Source: CAD feature listing. Evaluate the final solid. Frame: model axes, mm. Give positions to 0.01 mm unless a question says otherwise; leave off trailing zeros. Order: outer loops, then holes, each group sorted by start corner. A loop starts at its lowest first (then second) coordinate and runs counter-clockwise, first axis right, second up. Notation, with made-up numbers: M 74,11.5 L 123,11.5 A11 ccw 123,21.5 Z; hole C 78,13 d6. An arc over 180 degrees is marked long. Use CSV: the item, a comma, the result in double quotes. Start each with the question number.
1. Section query C-C, the plane y = -3.5. Return the cut outline in (x, z), plus the area to 3 significant figures.
2. Section query D-D, the plane x = -20. Return the cut outline in (y, z).
3. Line query: line 1 along X through (y, z) = (-1.25, 0.35); line 2 along Y through (x, z) = (30, 1.55); line 3 along X through (y, z) = (-0.5, 2.9). Output: solid intervals per line, ascending. Write a range as [from, to].
4. Pin query (flat end, axial travel): P1, Ø1.5, axis at y = 2, z = 1.5, coming from the -X side; P2, Ø2.5, axis at x = -20, y = 0, coming from the -Z side. Return the tip coordinate at first contact, or that it passes through.
5. Section query B-B, the plane z = 1.3. State how many separate pieces and enclosed holes the cut face has, plus the area to 3 significant figures.
6. Section query A-A, the plane x = 30. Return the cut outline in (y, z).
from build123d import *

# Parameters (mm, degrees)
SKETCH_1_W      = 60
SKETCH_1_H      = 12
SKETCH_1_R      = 1.5
EXTRUDE_1_DEPTH = 4
FILLET_1_R      = 6


with BuildPart() as part:
    # 草图1 → 凸台-拉伸1 (new body)
    with BuildSketch(Plane.XY):
        with Locations((5, 0)):
            Rectangle(SKETCH_1_W, SKETCH_1_H)
        with Locations((-20, 0)):
            Circle(SKETCH_1_R, mode=Mode.SUBTRACT)
        with Locations((30, 0)):
            Circle(SKETCH_1_R, mode=Mode.SUBTRACT)
    extrude(amount=EXTRUDE_1_DEPTH)

    # 圆角1
    fillet_1_edges = [part.edges().sort_by_distance(p)[0] for p in [
        (-25, -6, 2),
        (-25, 6, 2),
    ]]
    fillet(fillet_1_edges, radius=FILLET_1_R - 0.0001)  # a hair under: the kernel refuses the full size


solid = part.part
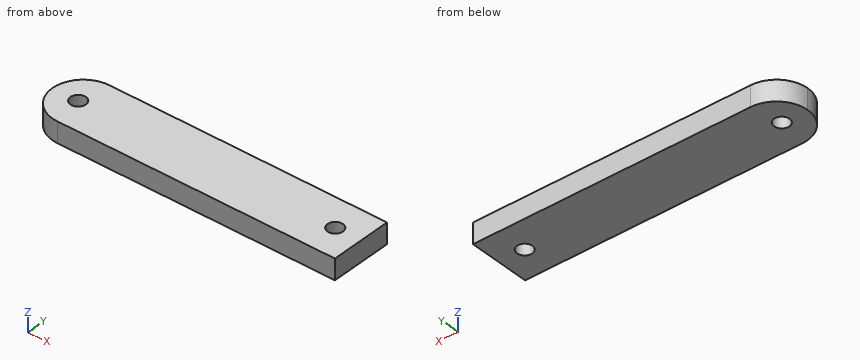
Result set:
1,outline,"M -23.87,0 L 35,0 L 35,4 L -23.87,4 Z"
1,area,"235 mm2"
2,outline,"M -5.92,0 L -1.5,0 L -1.5,4 L -5.92,4 Z; M 1.5,0 L 5.92,0 L 5.92,4 L 1.5,4 Z"
3,line 1,"[-24.87, -20.83], [-19.17, 29.17], [30.83, 35]"
3,line 2,"[-6, -1.5], [1.5, 6]"
3,line 3,"[-24.98, -21.41], [-18.59, 28.59], [31.41, 35]"
4,P1,"x = -24.87"
4,P2,"through"
5,separate pieces,"1"
5,enclosed holes,"2"
5,area,"690 mm2"
6,outline,"M -6,0 L -1.5,0 L -1.5,4 L -6,4 Z; M 1.5,0 L 6,0 L 6,4 L 1.5,4 Z"
